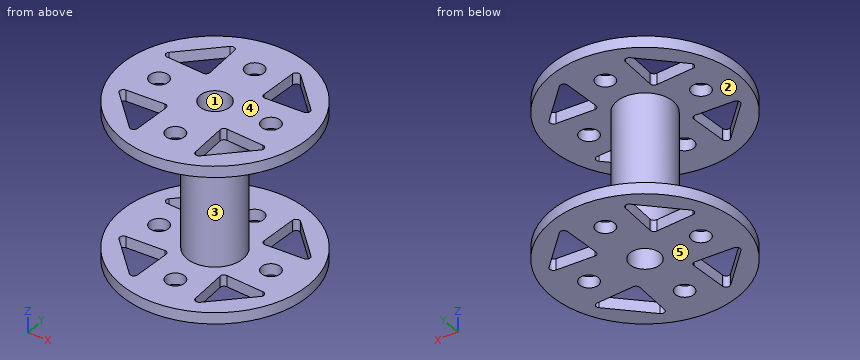
from build123d import *

# Parameters (mm, degrees)
CROQUIS1_R              = 7.5
CROQUIS1_R_2            = 4
SALIENTE_EXTRUIR1_DEPTH = 36
CROQUIS2_R              = 25
CROQUIS2_R_2            = 4
CROQUIS2_R_3            = 2.5
SALIENTE_EXTRUIR2_DEPTH = 3


with BuildPart() as part:
    # Croquis1 → Saliente-Extruir1 (new body)
    with BuildSketch(Plane.XY):
        Circle(CROQUIS1_R)
        Circle(CROQUIS1_R_2, mode=Mode.SUBTRACT)
    extrude(amount=SALIENTE_EXTRUIR1_DEPTH)

    # Croquis2 → Saliente-Extruir2 (add)
    with BuildSketch(Plane.XY.offset(36)):
        Circle(CROQUIS2_R)
        Circle(CROQUIS2_R_2, mode=Mode.SUBTRACT)
        with Locations((0, 15)):
            Circle(CROQUIS2_R_3, mode=Mode.SUBTRACT)
        with Locations((15, 0)):
            Circle(CROQUIS2_R_3, mode=Mode.SUBTRACT)
        with Locations((0, -15)):
            Circle(CROQUIS2_R_3, mode=Mode.SUBTRACT)
        with Locations((-15, 0)):
            Circle(CROQUIS2_R_3, mode=Mode.SUBTRACT)
        with BuildLine():
            Line((-19.027844597, 9.475344501), (-9.475344501, 19.027844597))
            ThreePointArc((-9.475344501, 19.027844597), (-8.409973952, 19.254358227), (-7.76961989, 18.373296649))
            Line((-7.76961989, 18.373296649), (-7.23892544, 8.290102103))
            ThreePointArc((-7.23892544, 8.290102103), (-7.530436489, 7.530436489), (-8.290102103, 7.23892544))
            Line((-8.290102103, 7.23892544), (-18.373296649, 7.76961989))
            ThreePointArc((-18.373296649, 7.76961989), (-19.254358227, 8.409973952), (-19.027844597, 9.475344501))
        make_face(mode=Mode.SUBTRACT)
        with BuildLine():
            Line((7.76961989, 18.373296649), (7.23892544, 8.290102103))
            ThreePointArc((7.23892544, 8.290102103), (7.530436489, 7.530436489), (8.290102103, 7.23892544))
            Line((8.290102103, 7.23892544), (18.373296649, 7.76961989))
            ThreePointArc((18.373296649, 7.76961989), (19.254358227, 8.409973952), (19.027844597, 9.475344501))
            Line((19.027844597, 9.475344501), (9.475344501, 19.027844597))
            ThreePointArc((9.475344501, 19.027844597), (8.409973952, 19.254358227), (7.76961989, 18.373296649))
        make_face(mode=Mode.SUBTRACT)
        with BuildLine():
            Line((18.373296649, -7.76961989), (8.290102103, -7.23892544))
            ThreePointArc((8.290102103, -7.23892544), (7.530436489, -7.530436489), (7.23892544, -8.290102103))
            Line((7.23892544, -8.290102103), (7.76961989, -18.373296649))
            ThreePointArc((7.76961989, -18.373296649), (8.409973952, -19.254358227), (9.475344501, -19.027844597))
            Line((9.475344501, -19.027844597), (19.027844597, -9.475344501))
            ThreePointArc((19.027844597, -9.475344501), (19.254358227, -8.409973952), (18.373296649, -7.76961989))
        make_face(mode=Mode.SUBTRACT)
        with BuildLine():
            Line((-7.76961989, -18.373296649), (-7.23892544, -8.290102103))
            ThreePointArc((-7.23892544, -8.290102103), (-7.530436489, -7.530436489), (-8.290102103, -7.23892544))
            Line((-8.290102103, -7.23892544), (-18.373296649, -7.76961989))
            ThreePointArc((-18.373296649, -7.76961989), (-19.254358227, -8.409973952), (-19.027844597, -9.475344501))
            Line((-19.027844597, -9.475344501), (-9.475344501, -19.027844597))
            ThreePointArc((-9.475344501, -19.027844597), (-8.409973952, -19.254358227), (-7.76961989, -18.373296649))
        make_face(mode=Mode.SUBTRACT)
    saliente_extruir2 = extrude(amount=SALIENTE_EXTRUIR2_DEPTH)

    # Simetría1: Saliente-Extruir2 across plane
    add(saliente_extruir2.mirror(Plane(origin=(0, 0, 18), x_dir=(1, 0, 0), z_dir=(0, 0, -1))))


solid = part.part
The listing builds one solid part. Answer for the finished solid, in the listing's coordinates (mm). Face numbers are marked on the shaded views. A direction names the side the tool comes from. Coordinates: 2 decimals unless noted, no trailing zeros. Loops run counter-clockwise (first coordinate to the right, second up) from the corner with the lowest first, then second, coordinate; pieces in that order, holes last.
1) Find section B-B on y = -20. Write down the section's boundary in (x, z).
2) Find the intervals of material crossed by L1, parallel to Y at x = 0, z = -0.6; L2, parallel to Z at x = -6.5, y = 21.5; L3, parallel to X at y = -8.5, z = 36.5, in increasing order.
3) Flat-ended cylindrical pins translate along their axes: pin 1 Ø6.5 at (x, y) = (-15, 0) entering from -Z; pin 2 Ø5 at (y, z) = (-18, 33) entering from +X; pin 3 Ø1.5 at (y, z) = (2.5, 18.5) entering from -X; pin 4 Ø12 at (y, z) = (8, 5.5) entering from +X. Find the tip coordinate at first contact, or state that the pin passes through.
4) A tool of negligible diameter and unlimited length cuts with its end or side. For the marked faces 1 and 2, from which of +Z, -Z, +X, -X, +Y, -Y can it reach the whole face along a straight path? Write none if from no direction.
5) Determine the mould class of the marked faces 3, 4 and 5 for opening direction Z: pulls with the +Z half, pulls with the -Z half, needs draft (parallel to the pull), parting line crosses it, or undercut.
6) Find section A-A on x = 0. Give the number of separate pieces and of enclosed holes in the cut face, then the cut area to 3 significant figures.
Values:
1. outline: (-15, -3) - (15, -3) - (15, 0) - (-15, 0) - close; (-15, 36) - (15, 36) - (15, 39) - (-15, 39) - close
2. L1: y = -25 to -17.5, -12.5 to -4, 4 to 12.5, 17.5 to 25
2. L2: z = -3 to 0, 36 to 39
2. L3: x = -23.51 to -19.28, -7.25 to 7.25, 19.28 to 23.51
3. pin 1: stops at z = -3
3. pin 2: passes through
3. pin 3: stops at x = -7.29
3. pin 4: stops at x = 24.36
4. face 1: +Z, -Z
4. face 2: none
5. face 3: undercut
5. face 4: pulls with the +Z half
5. face 5: pulls with the -Z half
6. separate pieces: 6
6. enclosed holes: 0
6. area: 444 mm2
